```python
from build123d import *

# Parameters (mm, degrees)
SKETCH1_R           = 4.65
BOSS_EXTRUDE1_DEPTH = 1
SKETCH2_R           = 4.65
SKETCH2_R_2         = 3.65
BOSS_EXTRUDE2_DEPTH = 11
BOSS_EXTRUDE3_DEPTH = 8
SKETCH4_W           = 9.6
SKETCH4_H           = 4.6
BOSS_EXTRUDE4_DEPTH = 0.3
SKETCH5_W           = 0.8
SKETCH5_H           = 0.5
CUT_EXTRUDE1_DEPTH  = 14.839888005
CUT_EXTRUDE2_DEPTH  = 14.735446844


with BuildPart() as part:
    # Sketch1 → Boss-Extrude1 (new body)
    with BuildSketch(Plane(origin=(0, 0, 0), x_dir=(1, 0, 0), z_dir=(0, 1, 0))):
        with Locations(Location((0, 0, 0), (0, 0, 270))):
            Circle(SKETCH1_R)
    extrude(amount=BOSS_EXTRUDE1_DEPTH)

    # Sketch2 → Boss-Extrude2 (add)
    with BuildSketch(Plane(origin=(0, 1, 0), x_dir=(1, 0, 0), z_dir=(0, 1, 0))):
        with Locations(Location((0, 0, 0), (0, 0, 270))):
            Circle(SKETCH2_R)
        with Locations(Location((0, 0, 0), (0, 0, 270))):
            Circle(SKETCH2_R_2, mode=Mode.SUBTRACT)
    extrude(amount=BOSS_EXTRUDE2_DEPTH)

    # Sketch3 → Boss-Extrude3 (add)
    with BuildSketch(Plane.XZ):
        with BuildLine():
            Line((0.35, -1.15), (-0.35, -1.15))
            ThreePointArc((-0.35, -1.15), (-1.5, 0), (-0.35, 1.15))
            Line((-0.35, 1.15), (0.35, 1.15))
            ThreePointArc((0.35, 1.15), (1.5, 0), (0.35, -1.15))
        make_face()
    extrude(amount=BOSS_EXTRUDE3_DEPTH)

    # Sketch4 → Boss-Extrude4 (add, symmetric)
    with BuildSketch(Plane.XY):
        with Locations((0, -4.7)):
            Rectangle(SKETCH4_W, SKETCH4_H)
    extrude(amount=BOSS_EXTRUDE4_DEPTH, both=True)

    # Sketch5 → Cut-Extrude1 (cut, through all)
    with BuildSketch(Plane(origin=(0, 0, -0.3), x_dir=(-1, 0, 0), z_dir=(0, 0, -1))):
        with Locations((-1.9, -2.65)):
            Rectangle(SKETCH5_W, SKETCH5_H)
        with Locations((-3.7, -2.65)):
            Rectangle(SKETCH5_W, SKETCH5_H)
        with Locations((3.7, -2.65)):
            Rectangle(SKETCH5_W, SKETCH5_H)
        with Locations((1.9, -2.65)):
            Rectangle(SKETCH5_W, SKETCH5_H)
        with Locations((1.9, -6.75)):
            Rectangle(SKETCH5_W, SKETCH5_H)
        with Locations((3.7, -6.75)):
            Rectangle(SKETCH5_W, SKETCH5_H)
        with Locations((-3.7, -6.75)):
            Rectangle(SKETCH5_W, SKETCH5_H)
        with Locations((-1.9, -6.75)):
            Rectangle(SKETCH5_W, SKETCH5_H)
    extrude(amount=-CUT_EXTRUDE1_DEPTH, mode=Mode.SUBTRACT)

    # Sketch6 → Cut-Extrude2 (cut, through all)
    with BuildSketch(Plane.XZ):
        with BuildLine():
            Line((-0.75, 1.5), (-2.25, 1.5))
            ThreePointArc((-2.25, 1.5), (-2.75, 2), (-2.25, 2.5))
            Line((-2.25, 2.5), (-0.75, 2.5))
            ThreePointArc((-0.75, 2.5), (-0.25, 2), (-0.75, 1.5))
        make_face()
        with BuildLine():
            Line((0.75, 1.5), (2.25, 1.5))
            ThreePointArc((2.25, 1.5), (2.75, 2), (2.25, 2.5))
            Line((2.25, 2.5), (0.75, 2.5))
            ThreePointArc((0.75, 2.5), (0.25, 2), (0.75, 1.5))
        make_face()
    extrude(amount=-CUT_EXTRUDE2_DEPTH, mode=Mode.SUBTRACT)


solid = part.part
```
Geometry: final body of the model. Coordinates: model frame, mm. A direction names the side the tool comes from. Coordinates: 2 decimals unless noted, no trailing zeros. Loops run counter-clockwise (first coordinate to the right, second up) from the corner with the lowest first, then second, coordinate; pieces in that order, holes last. Notation, with made-up numbers: (-15, -21) -> (8, -21) arc R21 ccw to (8, 15) -> close; hole circle Ø8 at (-11.5, 7.5). An arc over 180 degrees is marked (long way). Use a Markdown table: item, result. Add a question column.
(1) Section query D-D, the plane y = -1.5. Return loops of the section in (x, z), plus the area to 3 significant figures.
(2) Section query C-C, the plane x = -1.75. Return loops of the section in (y, z), plus the area to 3 significant figures.
(3) Pin query (flat end, axial travel): pin 1 Ø0.5 at (x, z) = (3, 0) entering from +Y; pin 2 Ø0.7 at (x, z) = (3.5, 0) entering from -Y; pin 3 Ø1 at (x, y) = (2.5, 0.5) entering from +Z. Return the tip coordinate at first contact, or that it passes through.
(4) Section query B-B, the plane y = 7.25. Return loops of the section in (x, z), plus the area to 3 significant figures.
(5) Access query for faces 1 (the flat face through (-3, -5, 0.3)), 2 (the cylindrical face through (-2.75, 0.49, 1.99)), 3 (the cylindrical face through (-1.4, 6.42, 3.37)), 4 (the flat face through (0, -8, 0)), 5 (the flat face through (3, -5, -0.3)). Directions: +Z, -Z, +X, -X, +Y, -Y. A direction counts if a zero-diameter tool reaches every point of the face in a straight line with its end or side. Return the directions, or none.
(6) Section query A-A, the plane z = 2. Return loops of the section in (x, y).
(7) Mould query, pull axis Z, two halves, no side actions, for faces 6 (the flat face through (3, -5, 0.3)), 7 (the cylindrical face through (0.25, 0.49, 2.01)), 8 (the flat face through (-4, 12, 0)). Classes: pulls with the +Z half, pulls with the -Z half, needs draft (parallel to the pull), parting line crosses it, or undercut.
(8) Line query: line 1 along X through (y, z) = (3.75, 0); line 2 along Y through (x, z) = (3, 0); line 3 along Y through (x, z) = (-2.5, 3.75). Output: solid intervals per line, ascending.
Answer:
| question | item | result |
|---|---|---|
| 1 | outline | (-0.35, -1.15) -> (0.35, -1.15) arc R1.15 ccw to (0.35, 1.15) -> (-0.35, 1.15) arc R1.15 ccw to start |
| 1 | area | 5.76 mm^2 |
| 2 | outline | (-6.5, -0.3) -> (-2.9, -0.3) -> (-2.9, 0.3) -> (-6.5, 0.3) -> close; (0, -4.31) -> (12, -4.31) -> (12, -3.2) -> (1, -3.2) -> (1, 1.5) -> (0, 1.5) -> close; (0, 2.5) -> (1, 2.5) -> (1, 3.2) -> (12, 3.2) -> (12, 4.31) -> (0, 4.31) -> close |
| 2 | area | 34.1 mm^2 |
| 3 | pin 1 | stops at y = 1 |
| 3 | pin 2 | stops at y = -7 |
| 3 | pin 3 | stops at z = 4.2 |
| 4 | outline | circle Ø9.3 at (0, 0); hole circle Ø7.3 at (0, 0) |
| 4 | area | 26.1 mm^2 |
| 5 | face 1 | +Z, -X, -Y |
| 5 | face 2 | +Y, -Y |
| 5 | face 3 | +Y |
| 5 | face 4 | +Z, -Z, +X, -X, -Y |
| 5 | face 5 | -Z, +X, -Y |
| 6 | outline | (-4.2, 0) -> (-2.75, 0) -> (-2.75, 1) -> (-3.05, 1) -> (-3.05, 12) -> (-4.2, 12) -> close; (-0.25, 0) -> (0.25, 0) -> (0.25, 1) -> (-0.25, 1) -> close; (2.75, 0) -> (4.2, 0) -> (4.2, 12) -> (3.05, 12) -> (3.05, 1) -> (2.75, 1) -> close |
| 7 | face 6 | pulls with the +Z half |
| 7 | face 7 | undercut |
| 7 | face 8 | needs draft |
| 8 | line 1 | x = -4.65 to -3.65, 3.65 to 4.65 |
| 8 | line 2 | y = -7 to -2.4, 0 to 1 |
| 8 | line 3 | y = 0 to 12 |
